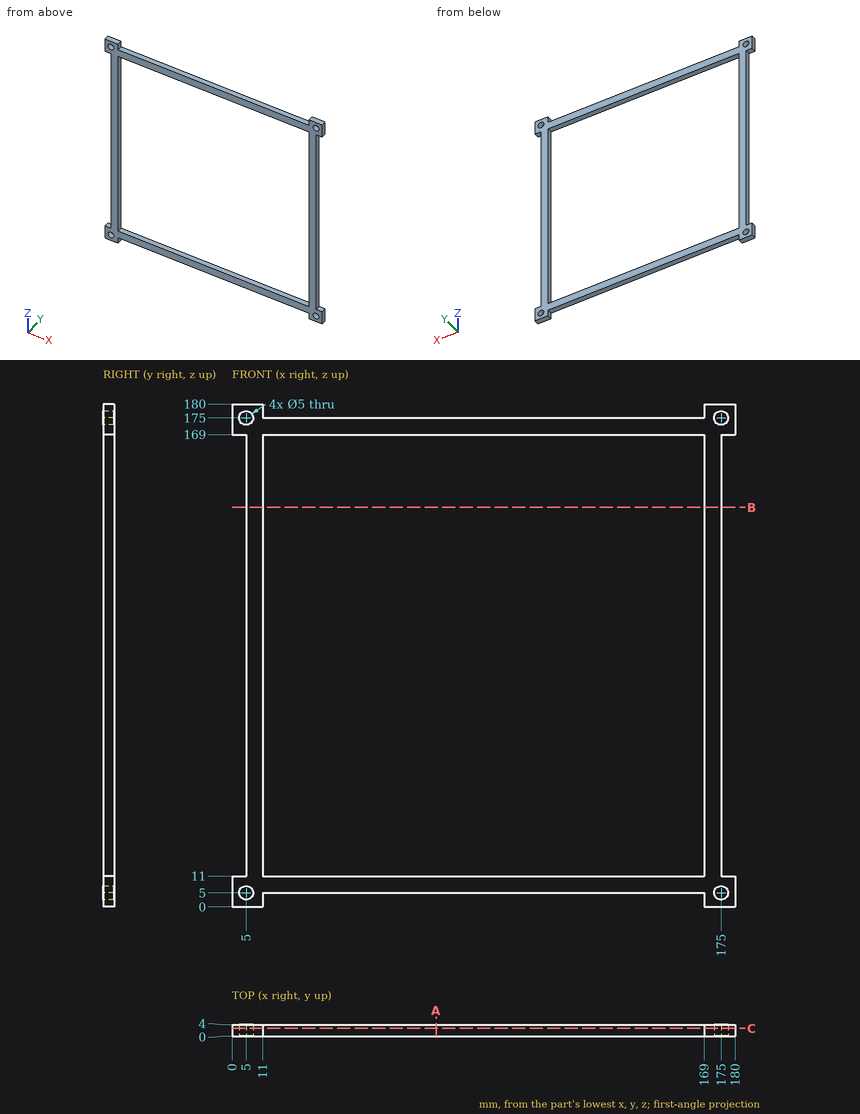
Here's the drawing with two shaded views (mm, measured from the low corner). I have some questions. Give positions to 0.01 mm unless a question says otherwise; leave off trailing zeros. Loops run counter-clockwise (first coordinate to the right, second up) from the corner with the lowest first, then second, coordinate; pieces in that order, holes last. Notation, with made-up numbers: (84.5, 60) - (130.5, 60) arc R20 cw to (130.5, 78) - close; hole circle Ø10 at (81.5, 4.5). An arc over 180 degrees is marked (long way). One line per item, written item: value.
(1) I need wall thicknesses on line 1 along Z through (x, y) = (126.5, 2.9). Which ranges of the line are inside material? Lowest first, please.
Verdict:
line 1: 5 to 11, 169 to 175
(2) If we section it at B-B, the plane z = 143: List the corners of the cut face in (x, y) for me, plus the area to 3 significant figures.
Verdict:
outline: (5, 0) - (11, 0) - (11, 4) - (5, 4) - close; (169, 0) - (175, 0) - (175, 4) - (169, 4) - close
area: 48.0 mm^2
(3) I'm going to push flat-ended pins straight in: pin 1 (1.2 mm diameter, centred on y = 1.5, z = 97.5, fed in from -X); pin 2 (2 mm diameter, centred on y = 2.5, z = 76, fed in from +X); pin 3 (1.2 mm diameter, centred on x = 120.5, y = 1, fed in from -Z). Where does each tip first touch, or does it pass through?
Verdict:
pin 1: x = 5
pin 2: x = 175
pin 3: z = 5
(4) If we section it at C-C, the plane y = 2.7: List the corners of the cut face in (x, z) for me.
Verdict:
outline: (0, 0) - (11, 0) - (11, 5) - (169, 5) - (169, 0) - (180, 0) - (180, 11) - (175, 11) - (175, 169) - (180, 169) - (180, 180) - (169, 180) - (169, 175) - (11, 175) - (11, 180) - (0, 180) - (0, 169) - (5, 169) - (5, 11) - (0, 11) - close; hole circle Ø5 at (5, 5); hole circle Ø5 at (5, 175); hole (11, 11) - (169, 11) - (169, 169) - (11, 169) - close; hole circle Ø5 at (175, 5); hole circle Ø5 at (175, 175)
(5) If we section it at A-A, the plane x = 73: List the corners of the cut face in (y, z) for me.
Verdict:
outline: (0, 5) - (4, 5) - (4, 11) - (0, 11) - close; (0, 169) - (4, 169) - (4, 175) - (0, 175) - close
